from build123d import *

# Parameters (mm, degrees)
SKETCH_R      = 4.5
SKETCH_R_2    = 2.8
PAD_DEPTH     = 4.5
SKETCH001_R   = 10
SKETCH001_R_2 = 1.65
PAD001_DEPTH  = 5
SKETCH002_R   = 1.65
POCKET_DEPTH  = 9.501


with BuildPart() as part:
    # Sketch → Pad (new body)
    with BuildSketch(Plane.XY):
        Circle(SKETCH_R)
        Circle(SKETCH_R_2, mode=Mode.SUBTRACT)
    extrude(amount=PAD_DEPTH)

    # Sketch001 (on Face4 of Pad) → Pad001 (join)
    with BuildSketch(Plane.XY.offset(4.5)):
        Circle(SKETCH001_R)
        Circle(SKETCH001_R_2, mode=Mode.SUBTRACT)
    extrude(amount=PAD001_DEPTH)

    # Sketch002 (on Face7 of Pad001) → Pocket (cut, through all)
    with BuildSketch(Plane.XY.offset(9.5)):
        with Locations((-7.3, 0)):
            Circle(SKETCH002_R)
        with Locations((0, -7.3)):
            Circle(SKETCH002_R)
        with Locations((0, 7.3)):
            Circle(SKETCH002_R)
        with Locations((7.3, 0)):
            Circle(SKETCH002_R)
    extrude(amount=-POCKET_DEPTH, mode=Mode.SUBTRACT)


solid = part.part
Source: CAD feature listing. Evaluate the final solid. Frame: model axes, mm. A direction names the side the tool comes from. Give positions to 0.01 mm unless a question says otherwise; leave off trailing zeros. Write each loop counter-clockwise with the first axis right and the second up, starting at its lowest first coordinate (ties: lowest second). Pieces come first, ordered by that corner, then holes. Notation, with made-up numbers: (-34, 88) - (2, 88) arc R22 ccw to (2, 125) - close; hole circle Ø3 at (53.25, 27.5). An arc over 180 degrees is marked (long way). Write item = value, one per line. Start each with the question number.
Q1. Draft query along Y for faces 1 (the cylindrical face through (-0.59, 4.46, 2.22)), 2 (the flat face through (0, 5, 4.5)), 3 (the cylindrical face through (-2.8, 0.1, 2.2)). Return one class per face: +Y half, -Y half, draft (parallel to the pull), parting line (faces both ways), or undercut.
Q2. Reachability of faces 4 (the flat face through (0, -2, 9.5)), 5 (the flat face through (0, -2, 4.5)) from +Z, -Z, +X, -X, +Y, -Y: full face, straight path, thin tool, end or side. Return the list, or none.
Q3. Cut plane C-C, the plane z = 3.75. Return loops of the section in (x, y).
Q4. Cut plane A-A, the plane x = 0. Return loops of the section in (y, z), then the cut area to 3 significant figures.
Q5. Material intervals for probe 1 along Y at (x, z) = (0, 8.4); probe 2 along Y at (x, z) = (0, 2.1); probe 3 along Z at (x, y) = (-5.5, 2.25), sorted ascending.
Q6. Pin query (flat end, axial travel): pin 1 Ø2 at (x, y) = (-6.5, 4.5) entering from -Z; pin 2 Ø4 at (x, z) = (-2.5, 1.5) entering from +Y; pin 3 Ø5 at (y, z) = (-3, 3.5) entering from +X. Return the tip coordinate at first contact, or that it passes through.
Q7. Cut plane D-D, the plane x = -8. Return loops of the section in (y, z).
Computed values:
q1.face_1 = parting line
q1.face_2 = draft
q1.face_3 = undercut
q2.face_4 = +Z, +X, -X, +Y, -Y
q2.face_5 = -Z
q3.outline = circle Ø9 at (0, 0); hole circle Ø5.6 at (0, 0)
q4.outline = (-10, 4.5) - (-8.95, 4.5) - (-8.95, 9.5) - (-10, 9.5) - close; (-5.65, 4.5) - (-4.5, 4.5) - (-4.5, 0) - (-2.8, 0) - (-2.8, 4.5) - (-1.65, 4.5) - (-1.65, 9.5) - (-5.65, 9.5) - close; (1.65, 4.5) - (2.8, 4.5) - (2.8, 0) - (4.5, 0) - (4.5, 4.5) - (5.65, 4.5) - (5.65, 9.5) - (1.65, 9.5) - close; (8.95, 4.5) - (10, 4.5) - (10, 9.5) - (8.95, 9.5) - close
q4.area = 65.8 mm²
q5.probe_1 = -10 to -8.95, -5.65 to -1.65, 1.65 to 5.65, 8.95 to 10
q5.probe_2 = -4.5 to -2.8, 2.8 to 4.5
q5.probe_3 = 4.5 to 9.5
q6.pin_1 = 4.5
q6.pin_2 = 4.47
q6.pin_3 = 9.97
q7.outline = (-6, 4.5) - (-1.49, 4.5) - (-1.49, 9.5) - (-6, 9.5) - close; (1.49, 4.5) - (6, 4.5) - (6, 9.5) - (1.49, 9.5) - close
